Source: three-view drawing plus pictorial views. Frame: mm from the lowest corner of the part. Round coordinates to 2 decimals unless told otherwise and drop trailing zeros. Loops run counter-clockwise (first coordinate to the right, second up) from the corner with the lowest first, then second, coordinate; pieces in that order, holes last. Notation, with made-up numbers: M 16.5,84 L 26.5,84 A23 cw 26.5,92 Z; hole C -31.75,81 d10. An arc over 180 degrees is marked long. Return JSON: item names as keys, results as strings. Group by question number.
1) Material intervals for line 1 (Z direction, x = 1.05, y = 3); line 2 (Z direction, x = 1, y = 3.25), sorted ascending. Write a range as from..to.
2) Contact query for flat-ended pins moving along their axis: P1, Ø1.5, axis at y = 3.89, z = 3.89, coming from the +X side; P2, Ø1, axis at x = 0.5, y = 6, coming from the +Z side; P3, Ø4, axis at y = 5, z = 5, coming from the -X side. Output: stop coordinate, or through.
3) Section A-A (x = 1.55). Output: boundary loops of the cut face in (y, z), plus the area to 3 significant figures.
4) Mould query, pull axis Y, two halves, no side actions, for the marked faces 1, 2, 3 and 4. Classes: +Y half, -Y half, draft (parallel to the pull), parting line (faces both ways), or undercut.
5) Section B-B (y = 1). Output: boundary loops of the cut face in (x, z), plus the area to 3 significant figures.
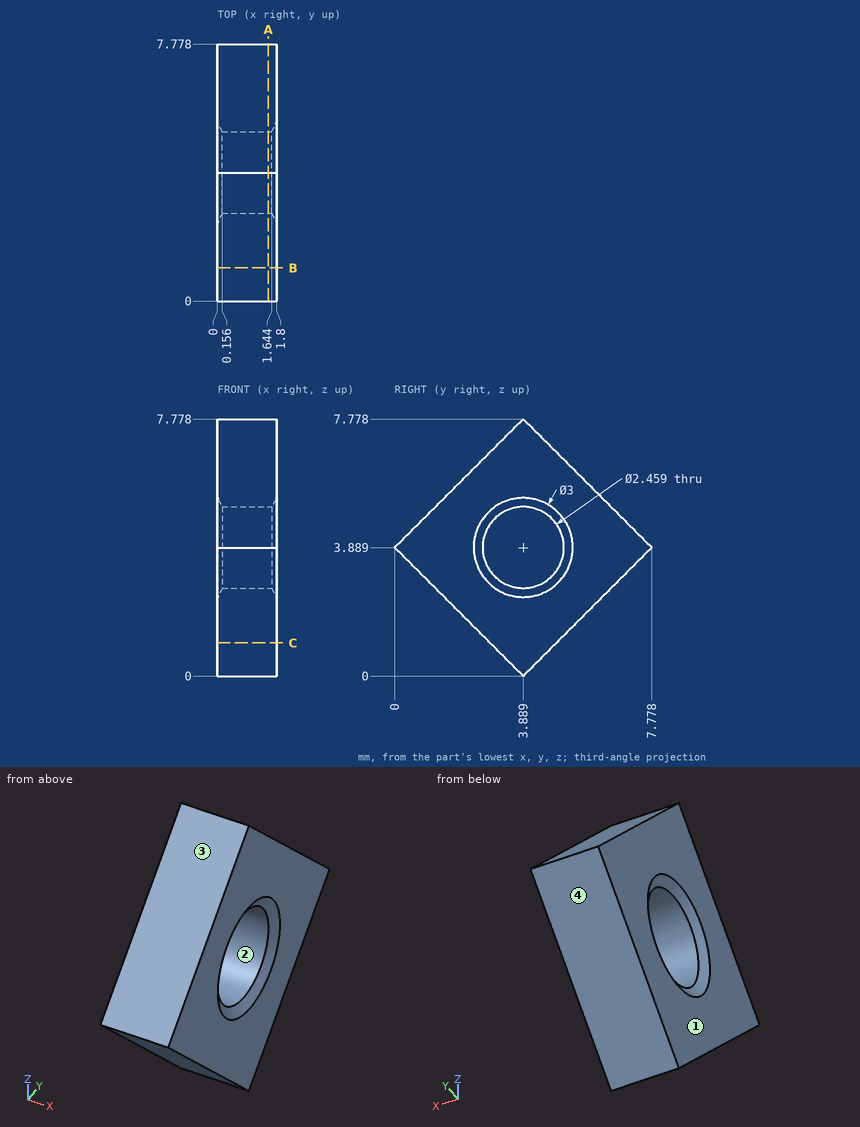
Returned:
{
 "1": {"line 1": "z = 0.89..3.04, 4.74..6.89", "line 2": "z = 0.64..2.84, 4.94..7.14"},
 "2": {"P1": "passes through", "P2": "stops at z = 6.17", "P3": "stops at x = 0"},
 "3": {"outline": "M 0,3.89 L 3.89,0 L 7.78,3.89 L 3.89,7.78 Z; hole C 3.89,3.89 d2.46", "area": "25.5 mm^2"},
 "4": {"face 1": "draft", "face 2": "undercut", "face 3": "-Y half", "face 4": "+Y half"},
 "5": {"outline": "M 0,2.89 L 1.8,2.89 L 1.8,4.89 L 0,4.89 Z", "area": "3.60 mm^2"}
}
